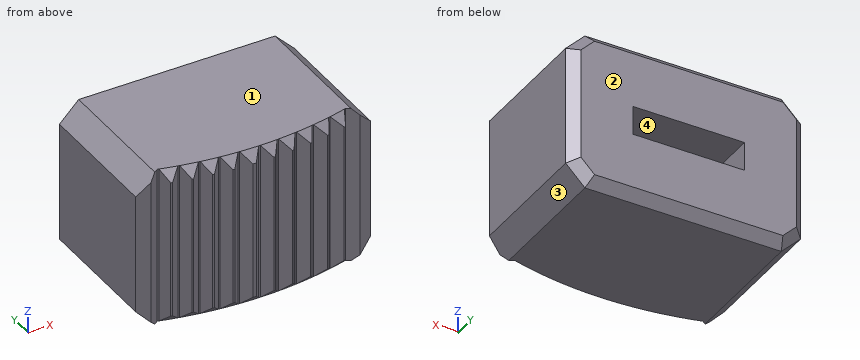
```python
from build123d import *

# Parameters (mm, degrees)
F1_DEPTH = 4.1
F3_DEPTH = 0.75
F4_SIZE  = 1
F5_SIZE  = 0.5
F6_SIZE  = 0.5


# Not quite as in the source:
# - ends of sketch curves that miss each other by under 0.0002 mm in the source are joined


with BuildPart() as f1:
    # F0 (on Top) → F1 (new body, symmetric)
    with BuildSketch(Plane.XY):
        with BuildLine():
            Line((-6.1, 4.15), (-6.1, -3.15))
            ThreePointArc((-6.1, -3.15), (-5.7635565841, -3.2598963663), (-5.425135, -3.363541))
            Line((-5.425135, -3.363541), (-4.893695, -2.994868))
            Line((-4.893695, -2.994868), (-4.8153280581, -3.0160501894))
            Line((-4.8153280581, -3.0160501894), (-4.5419790581, -3.6022481894))
            ThreePointArc((-4.5419790581, -3.6022481894), (-4.5004913685, -3.6123533808), (-4.4589811968, -3.62236582))
            Line((-4.4589811968, -3.62236582), (-3.9475651968, -3.22638582))
            Line((-3.9475651968, -3.22638582), (-3.8681969582, -3.2434357798))
            Line((-3.8681969582, -3.2434357798), (-3.5645439582, -3.8145247798))
            ThreePointArc((-3.5645439582, -3.8145247798), (-3.5225838002, -3.822444913), (-3.4806060449, -3.8302712423))
            Line((-3.4806060449, -3.8302712423), (-2.9906150449, -3.4080672423))
            Line((-2.9906150449, -3.4080672423), (-2.9104630974, -3.4209427155))
            Line((-2.9104630974, -3.4209427155), (-2.5773370974, -3.9753557155))
            ThreePointArc((-2.5773370974, -3.9753557155), (-2.5350204133, -3.9810689039), (-2.4926910656, -3.9866874981))
            Line((-2.4926910656, -3.9866874981), (-2.0254680656, -3.5394184981))
            Line((-2.0254680656, -3.5394184981), (-1.9447520573, -3.5480806887))
            Line((-1.9447520573, -3.5480806887), (-1.5830670573, -4.0842996887))
            ThreePointArc((-1.5830670573, -4.0842996887), (-1.5405093729, -4.0877903631), (-1.4979439929, -4.0911859103))
            Line((-1.4979439929, -4.0911859103), (-1.0547689929, -3.6200769103))
            Line((-1.0547689929, -3.6200769103), (-0.9737100092, -3.624502302))
            Line((-0.9737100092, -3.624502302), (-0.5844580092, -4.141058302))
            ThreePointArc((-0.5844580092, -4.141058302), (-0.5001103826, -4.1434534303), (-0.415753, -4.1454759956))
            Line((-0.415753, -4.1454759956), (0, -3.6499999956))
            Line((0, -3.6499999956), (0.0811800024, -3.649823093))
            Line((0.0811800024, -3.649823093), (0.4990910024, -4.143480093))
            ThreePointArc((0.4990910024, -4.143480093), (0.541775859, -4.1423168954), (0.5844580091, -4.1410582978))
            Line((0.5844580091, -4.1410582978), (0.9737110091, -3.6245022978))
            Line((0.9737110091, -3.6245022978), (1.0547699921, -3.6200768997))
            Line((1.0547699921, -3.6200768997), (1.4979439921, -4.0911858997))
            ThreePointArc((1.4979439921, -4.0911858997), (1.5405098686, -4.087790312), (1.5830680495, -4.084299595))
            Line((1.5830680495, -4.084299595), (1.9447520495, -3.548080595))
            Line((1.9447520495, -3.548080595), (2.0254690462, -3.5394183512))
            Line((2.0254690462, -3.5394183512), (2.4926920462, -3.9866873512))
            ThreePointArc((2.4926920462, -3.9866873512), (2.5350213933, -3.9810687545), (2.5773380767, -3.9753555637))
            Line((2.5773380767, -3.9753555637), (2.9104640767, -3.4209425637))
            Line((2.9104640767, -3.4209425637), (2.9906160072, -3.4080670388))
            Line((2.9906160072, -3.4080670388), (3.4806070072, -3.8302710388))
            ThreePointArc((3.4806070072, -3.8302710388), (3.5225842788, -3.8224447977), (3.5645439535, -3.814524755))
            Line((3.5645439535, -3.814524755), (3.8681969535, -3.243435755))
            Line((3.8681969535, -3.243435755), (3.947566135, -3.2263855622))
            Line((3.947566135, -3.2263855622), (4.458982135, -3.6223655622))
            ThreePointArc((4.458982135, -3.6223655622), (4.5004922999, -3.6123531221), (4.5419799828, -3.6022479298))
            Line((4.5419799828, -3.6022479298), (4.8153289828, -3.0160499298))
            Line((4.8153289828, -3.0160499298), (4.893695989, -2.994867963))
            Line((4.893695989, -2.994867963), (5.425134989, -3.363540963))
            ThreePointArc((5.425134989, -3.363540963), (5.7635565104, -3.2598963467), (6.0999999321, -3.1500002293))
            Line((6.0999999321, -3.1500002293), (6.1, 4.15))
            Line((6.1, 4.15), (-6.1, 4.15))
        make_face()
    extrude(amount=F1_DEPTH, both=True)

    # F2 (on Top) → F3 (cut, symmetric)
    with BuildSketch(Plane.XY):
        with BuildLine():
            Line((2.9, 4.15), (-2.9, 4.15))
            Line((-2.9, 4.15), (-2.9, -0.85))
            ThreePointArc((-2.9, -0.85), (0, -1.85), (2.9, -0.85))
            Line((2.9, -0.85), (2.9, 4.15))
        make_face()
    extrude(amount=F3_DEPTH, both=True, mode=Mode.SUBTRACT)

    # F4
    f4_edges = [f1.edges().sort_by_distance(p)[0] for p in [
        (6.1, 0.5, -4.1),
        (-6.1, 0.5, -4.1),
        (-6.1, 0.5, 4.1),
        (6.1, 0.5, 4.1),
    ]]
    chamfer(f4_edges, length=F4_SIZE)

    # F5
    f5_edges = [f1.edges().sort_by_distance(p)[0] for p in [
        (0, 4.15, -4.1),
        (-5.6, 4.15, -3.6),
        (-6.1, 4.15, 0),
        (5.6, 4.15, -3.6),
        (6.1, 4.15, 0),
        (5.6, 4.15, 3.6),
        (0, 4.15, 4.1),
        (-5.6, 4.15, 3.6),
    ]]
    chamfer(f5_edges, length=F5_SIZE)

    # F6
    f6_edges = [f1.edges().sort_by_distance(p)[0] for p in [
        (-2.53502, -3.981069, -4.1),
        (-3.522584, -3.822445, -4.1),
        (-4.500491, -3.612353, -4.1),
        (-1.540509, -4.08779, -4.1),
        (-0.50011, -4.143453, -4.1),
        (0.541776, -4.142317, -4.1),
        (1.54051, -4.08779, -4.1),
        (2.535021, -3.981069, -4.1),
        (3.522584, -3.822445, -4.1),
        (4.500492, -3.612353, -4.1),
        (-4.500491, -3.612353, 4.1),
        (-3.522584, -3.822445, 4.1),
        (-2.53502, -3.981069, 4.1),
        (-1.540509, -4.08779, 4.1),
        (-0.50011, -4.143453, 4.1),
        (0.541776, -4.142317, 4.1),
        (1.54051, -4.08779, 4.1),
        (2.535021, -3.981069, 4.1),
        (3.522584, -3.822445, 4.1),
        (4.500492, -3.612353, 4.1),
    ]]
    chamfer(f6_edges, length=F6_SIZE)


solid = f1.part
```
Input: part model. Units: mm. Frame: model coordinates. Face numbers are marked on the shaded views. Coordinates: 2 decimals unless noted, no trailing zeros. Loops run counter-clockwise (first coordinate to the right, second up) from the corner with the lowest first, then second, coordinate; pieces in that order, holes last.
Q1. Section B-B, the plane y = 2.5. Return the cut outline in (x, z), and give its area (3 significant figures).
Results are:
outline: (-6.1, -3.1) - (-5.1, -4.1) - (5.1, -4.1) - (6.1, -3.1) - (6.1, 3.1) - (5.1, 4.1) - (-5.1, 4.1) - (-6.1, 3.1) - close; hole (-2.9, -0.75) - (2.9, -0.75) - (2.9, 0.75) - (-2.9, 0.75) - close
area: 89.3 mm2
Q2. Section A-A, the plane y = -2.5. Return the cut outline in (x, z).
Results are:
outline: (-6.1, -3.1) - (-5.1, -4.1) - (5.1, -4.1) - (6.1, -3.1) - (6.1, 3.1) - (5.1, 4.1) - (-5.1, 4.1) - (-6.1, 3.1) - close
Q3. Contact query for a flat-ended pin moving along its axis: pin 1 (3 mm diameter, centred on x = 3, z = -2.5, fed in from -Y). Output: stop coordinate, or through.
Results are:
pin 1: stops at y = -4.09
Q4. Section C-C, the plane x = -5.25. Return the cut outline in (y, z), and give its area (3 significant figures).
Results are:
outline: (-3.24, -3.95) - (3.65, -3.95) - (4.15, -3.24) - (4.15, 3.24) - (3.65, 3.95) - (-3.24, 3.95) - close
area: 58.0 mm2
Q5. Mould query, pull axis Z, two halves, no side actions, for the marked faces 1, 2, 3 and 4. Classes: +Z half, -Z half, draft (parallel to the pull), parting line (faces both ways), or undercut.
Results are:
face 1: +Z half
face 2: draft
face 3: -Z half
face 4: undercut
Q6. Line query: line 1 along Z through (x, y) = (1.75, -1); line 2 along Z through (x, y) = (-5.25, 2.5); line 3 along Y through (x, z) = (-0.25, -3.25). Output: solid intervals per line, ascending.
Results are:
line 1: z = -4.1 to -0.75, 0.75 to 4.1
line 2: z = -3.95 to 3.95
line 3: y = -3.95 to 4.15
